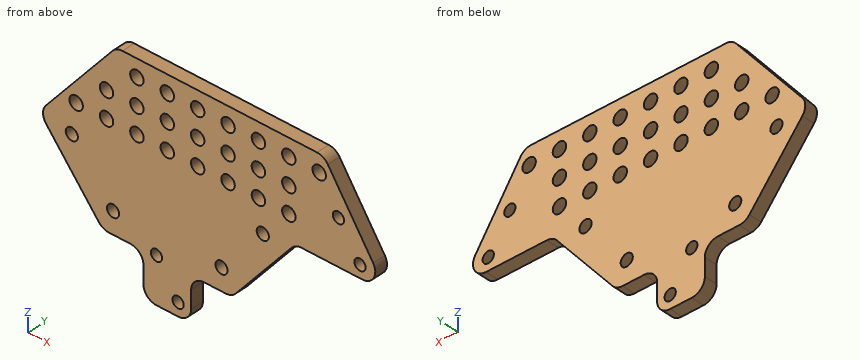
from build123d import *

# Parameters (mm, degrees)
SKETCH_1_R      = 1.55
SKETCH_1_R_2    = 1.4
SKETCH_1_R_3    = 1.3
EXTRUDE_1_DEPTH = 3
FILLET_6_R      = 3
FILLET_7_R      = 3


with BuildPart() as part:
    # 草图1 → 凸台-拉伸1 (new body)
    with BuildSketch(Plane(origin=(0, 0, 0), x_dir=(1, 0, 0), z_dir=(0, 1, 0))):
        Polygon((5.5, 26.649748742), (-5.5, 26.649748742), (-5.5, 16.608186766), (-14.869017707, 16.608186766), (-29.51289706, -1.285380235), (-11.741914225, -23), (36.109047815, -23), (50.51289706, -1.285380235), (31.937783614, -1.285380235), (29.51289706, -1.285380235), (14.869017707, 16.608186766), (5.5, 16.608186766), align=None)
        with Locations(Location((0, -19.02478316, 0), (0, 0, 270))):
            Circle(SKETCH_1_R, mode=Mode.SUBTRACT)
        with Locations(Location((7, -19.02478316, 0), (0, 0, 270))):
            Circle(SKETCH_1_R, mode=Mode.SUBTRACT)
        with Locations(Location((14, -19.02478316, 0), (0, 0, 270))):
            Circle(SKETCH_1_R, mode=Mode.SUBTRACT)
        with Locations(Location((21, -19.02478316, 0), (0, 0, 270))):
            Circle(SKETCH_1_R, mode=Mode.SUBTRACT)
        with Locations(Location((28, -19.02478316, 0), (0, 0, 270))):
            Circle(SKETCH_1_R, mode=Mode.SUBTRACT)
        with Locations(Location((35, -19.02478316, 0), (0, 0, 270))):
            Circle(SKETCH_1_R, mode=Mode.SUBTRACT)
        with Locations(Location((-7, -19.02478316, 0), (0, 0, 270))):
            Circle(SKETCH_1_R, mode=Mode.SUBTRACT)
        with Locations(Location((-14, -13.02478316, 0), (0, 0, 270))):
            Circle(SKETCH_1_R, mode=Mode.SUBTRACT)
        with BuildLine():
            ThreePointArc((-8.55, -13.02478316), (-7, -11.47478316), (-5.45, -13.02478316))
            ThreePointArc((-5.45, -13.02478316), (-7, -14.57478316), (-8.55, -13.02478316))
        make_face(mode=Mode.SUBTRACT)
        with Locations(Location((0, -13.02478316, 0), (0, 0, 270))):
            Circle(SKETCH_1_R, mode=Mode.SUBTRACT)
        with Locations(Location((7, -13.02478316, 0), (0, 0, 270))):
            Circle(SKETCH_1_R, mode=Mode.SUBTRACT)
        with Locations(Location((-21, -7.02478316, 0), (0, 0, 270))):
            Circle(SKETCH_1_R, mode=Mode.SUBTRACT)
        with Locations(Location((-14, -7.02478316, 0), (0, 0, 270))):
            Circle(SKETCH_1_R, mode=Mode.SUBTRACT)
        with Locations(Location((-7, -7.02478316, 0), (0, 0, 270))):
            Circle(SKETCH_1_R, mode=Mode.SUBTRACT)
        with Locations(Location((-22, 0, 0), (0, 0, 270))):
            Circle(SKETCH_1_R_2, mode=Mode.SUBTRACT)
        with Locations(Location((0, -7.02478316, 0), (0, 0, 270))):
            Circle(SKETCH_1_R, mode=Mode.SUBTRACT)
        with Locations(Location((7, -7.02478316, 0), (0, 0, 270))):
            Circle(SKETCH_1_R, mode=Mode.SUBTRACT)
        with Locations(Location((14, -13.02478316, 0), (0, 0, 270))):
            Circle(SKETCH_1_R, mode=Mode.SUBTRACT)
        with Locations(Location((21, -13.02478316, 0), (0, 0, 270))):
            Circle(SKETCH_1_R, mode=Mode.SUBTRACT)
        with Locations(Location((28, -13.02478316, 0), (0, 0, 270))):
            Circle(SKETCH_1_R, mode=Mode.SUBTRACT)
        with Locations(Location((39.429198074, -11.654622417, 0), (0, 0, 270))):
            Circle(SKETCH_1_R_3, mode=Mode.SUBTRACT)
        with Locations(Location((14, -7.02478316, 0), (0, 0, 270))):
            Circle(SKETCH_1_R, mode=Mode.SUBTRACT)
        with Locations(Location((21, -7.02478316, 0), (0, 0, 270))):
            Circle(SKETCH_1_R, mode=Mode.SUBTRACT)
        with Locations(Location((28, -7.02478316, 0), (0, 0, 270))):
            Circle(SKETCH_1_R, mode=Mode.SUBTRACT)
        with Locations(Location((22, 0, 0), (0, 0, 270))):
            Circle(SKETCH_1_R_2, mode=Mode.SUBTRACT)
        with Locations(Location((44.404135259, -4.154622417, 0), (0, 0, 270))):
            Circle(SKETCH_1_R_3, mode=Mode.SUBTRACT)
        with Locations(Location((-12.5, 11.608186766, 0), (0, 0, 270))):
            Circle(SKETCH_1_R_2, mode=Mode.SUBTRACT)
        with Locations(Location((-2.487468593, 16.149748742, 0), (0, 0, 270))):
            Circle(SKETCH_1_R_3, mode=Mode.SUBTRACT)
        with Locations(Location((2.487468593, 23.649748742, 0), (0, 0, 270))):
            Circle(SKETCH_1_R_3, mode=Mode.SUBTRACT)
        with Locations(Location((12.5, 11.608186766, 0), (0, 0, 270))):
            Circle(SKETCH_1_R_2, mode=Mode.SUBTRACT)
    extrude(amount=EXTRUDE_1_DEPTH)

    # 圆角6
    fillet_6_edges = [part.edges().sort_by_distance(p)[0] for p in [
        (-5.5, 1.5, -16.608186766),
        (5.5, 1.5, -16.608186766),
    ]]
    fillet(fillet_6_edges, radius=FILLET_6_R)

    # 圆角7
    fillet_7_edges = [part.edges().sort_by_distance(p)[0] for p in [
        (14.869017707, 1.5, -16.608186766),
        (29.51289706, 1.5, 1.285380235),
        (50.51289706, 1.5, 1.285380235),
        (36.109047815, 1.5, 23),
        (-11.741914225, 1.5, 23),
        (-29.51289706, 1.5, 1.285380235),
        (-14.869017707, 1.5, -16.608186766),
        (-5.5, 1.5, -26.649748742),
        (5.5, 1.5, -26.649748742),
    ]]
    fillet(fillet_7_edges, radius=FILLET_7_R)


solid = part.part
Source: CAD feature listing. Evaluate the final solid. Frame: model axes, mm. Round coordinates to 2 decimals unless told otherwise and drop trailing zeros. Loops run counter-clockwise (first coordinate to the right, second up) from the corner with the lowest first, then second, coordinate; pieces in that order, holes last. Notation, with made-up numbers: (-33.75, 84.25) -> (2.25, 84.25) arc R14 ccw to (2.25, 99.25) -> close; hole circle Ø4 at (-10, 23). An arc over 180 degrees is marked (long way). Answer as a JSON object with one key per item and string values. Group by question number.
Q1. Section query A-A (x = 0). Output: boundary loops of the cut face in (y, z), plus the area to 3 significant figures.
Q2. Ray query, line 1 (X direction, y = 2.05, z = 0.5); line 2 (X direction, y = 1.9, z = 0); line 3 (Z direction, x = -0.5, y = 1.1). Return the intervals inside material, ascending. Write a range as from..to.
Q3. Contact query for flat-ended pins moving along their axis: P1, Ø4, axis at x = 0, z = 19.02, coming from the +Y side; P2, Ø1.5, axis at x = 39, y = 1.5, coming from the -Z side; P3, Ø0.9, axis at y = 2, z = -22, coming from the +X side; P4, Ø1.5, axis at x = -11.5, y = 1, coming from the -Z side. Output: stop coordinate, or through.
Q4. Section query C-C (y = 2.4). State how many separate pieces and enclosed holes the cut face has, plus the area to 3 significant figures.
Q5. Section query B-B (z = -6.5). Output: boundary loops of the cut face in (x, y), plus the area to 3 significant figures.
Completed:
{
 "1": {"outline": "(0, -26.65) -> (3, -26.65) -> (3, 5.47) -> (0, 5.47) -> close; (0, 8.57) -> (3, 8.57) -> (3, 11.47) -> (0, 11.47) -> close; (0, 14.57) -> (3, 14.57) -> (3, 17.47) -> (0, 17.47) -> close; (0, 20.57) -> (3, 20.57) -> (3, 23) -> (0, 23) -> close", "area": "121 mm²"},
 "2": {"line 1": "-28.53..-23.31, -20.69..20.69, 23.31..28.91", "line 2": "-28.35..-23.4, -20.6..20.6, 23.4..28.46", "line 3": "-26.65..5.56, 8.49..11.56, 14.49..17.56, 20.49..23"},
 "3": {"P1": "y = 3", "P2": "z = 1.29", "P3": "x = 5.5", "P4": "z = -16.61"},
 "4": {"separate pieces": "1", "enclosed holes": "30", "area": "2,070 mm²"},
 "5": {"outline": "(-23.14, 0) -> (23.14, 0) -> (23.14, 3) -> (-23.14, 3) -> close", "area": "139 mm²"}
}
